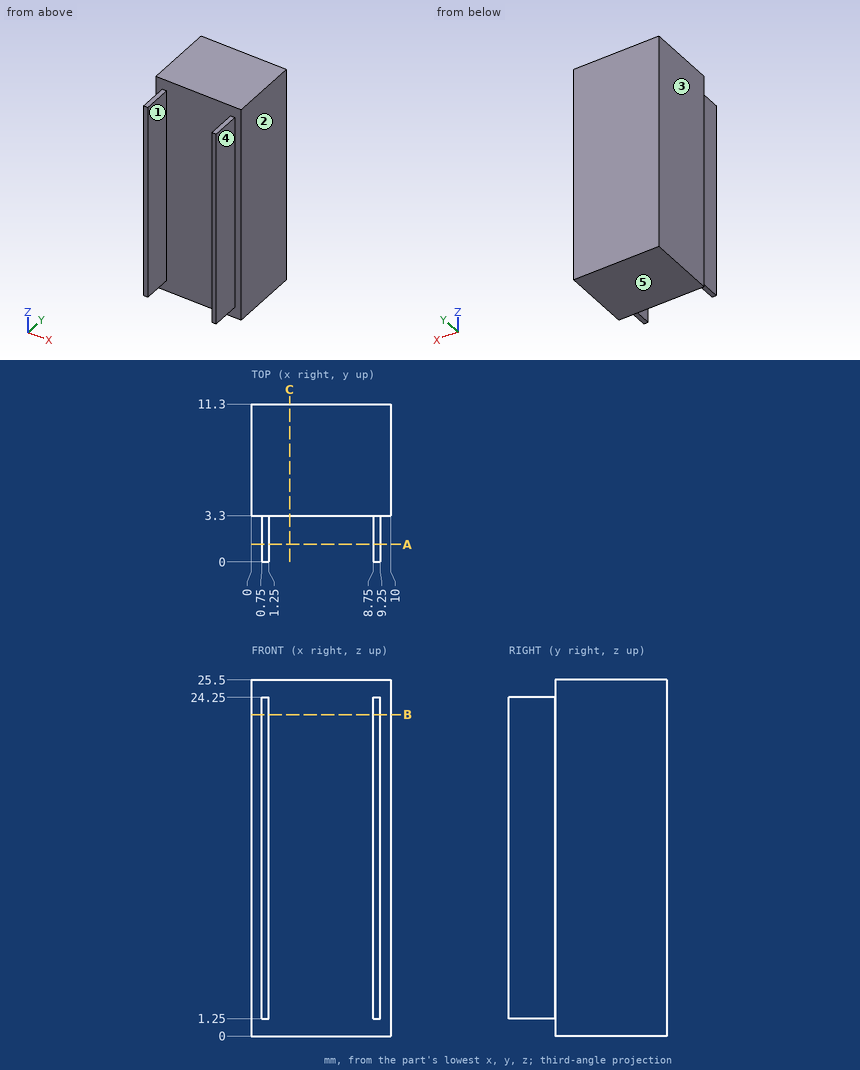
The drawing under review shows one solid part. Ordinate dimensions are in mm from its lowest x, y, z. A direction names the side the tool comes from. Coordinates: 2 decimals unless noted, no trailing zeros. Order: outer loops, then holes, each group sorted by start corner. A loop starts at its lowest first (then second) coordinate and runs counter-clockwise, first axis right, second up. Notation, with made-up numbers: (-7.5, -25.75) -> (1.5, -25.75) arc R22 cw to (1.5, -9.75) -> close; hole circle Ø3 at (23.5, -24). An arc over 180 degrees is marked (long way). Answer in a Markdown table with one row per item. Add a question column.
Item 1: Clearance check with flat-ended pins moving along their axes: pin 1 (0.6 mm diameter, centred on x = 1, y = 1, fed in from -Z); pin 2 (1 mm diameter, centred on y = 2, z = 12, fed in from -X); pin 3 (1.7 mm diameter, centred on y = 2, z = 9.5, fed in from +X). State where each tip first meets the part, or that it passes through.
Item 2: We need section A-A on y = 1.25. Write out the cut boundary in (x, z), plus the area to 3 significant figures.
Item 3: We need section B-B on z = 23. Write out the cut boundary in (x, y).
Item 4: Mouldability with a two-part tool opening along X and no side actions: class the marked faces 1, 2 and 3 as +X half, -X half, draft (parallel to the pull), parting line (faces both ways), or undercut.
Item 5: To check wall thickness, follow probe 1 along X at (y, z) = (1.5, 1.5); probe 2 along Y at (x, z) = (5.75, 6). State the ranges of each line that lie inside material, in increasing order.
Item 6: We need section C-C on x = 2.75. Write out the cut boundary in (y, z).
Item 7: Machinability: for the marked faces 4 and 5, which of the approach directions +Z, -Z, +X, -X, +Y, -Y give a long, thin tool a straight path to every point of the face, cutting with its end or side? Answer none if there is none.
Final values:
| question | item | result |
|---|---|---|
| 1 | pin 1 | stops at z = 1.25 |
| 1 | pin 2 | stops at x = 0.75 |
| 1 | pin 3 | stops at x = 9.25 |
| 2 | outline | (0.75, 1.25) -> (1.25, 1.25) -> (1.25, 24.25) -> (0.75, 24.25) -> close; (8.75, 1.25) -> (9.25, 1.25) -> (9.25, 24.25) -> (8.75, 24.25) -> close |
| 2 | area | 23.0 mm2 |
| 3 | outline | (0, 3.3) -> (0.75, 3.3) -> (0.75, 0) -> (1.25, 0) -> (1.25, 3.3) -> (8.75, 3.3) -> (8.75, 0) -> (9.25, 0) -> (9.25, 3.3) -> (10, 3.3) -> (10, 11.3) -> (0, 11.3) -> close |
| 4 | face 1 | undercut |
| 4 | face 2 | +X half |
| 4 | face 3 | -X half |
| 5 | probe 1 | x = 0.75 to 1.25, 8.75 to 9.25 |
| 5 | probe 2 | y = 3.3 to 11.3 |
| 6 | outline | (3.3, 0) -> (11.3, 0) -> (11.3, 25.5) -> (3.3, 25.5) -> close |
| 7 | face 4 | +Z, -Z, +X, -Y |
| 7 | face 5 | -Z, +X, -X, +Y, -Y |
